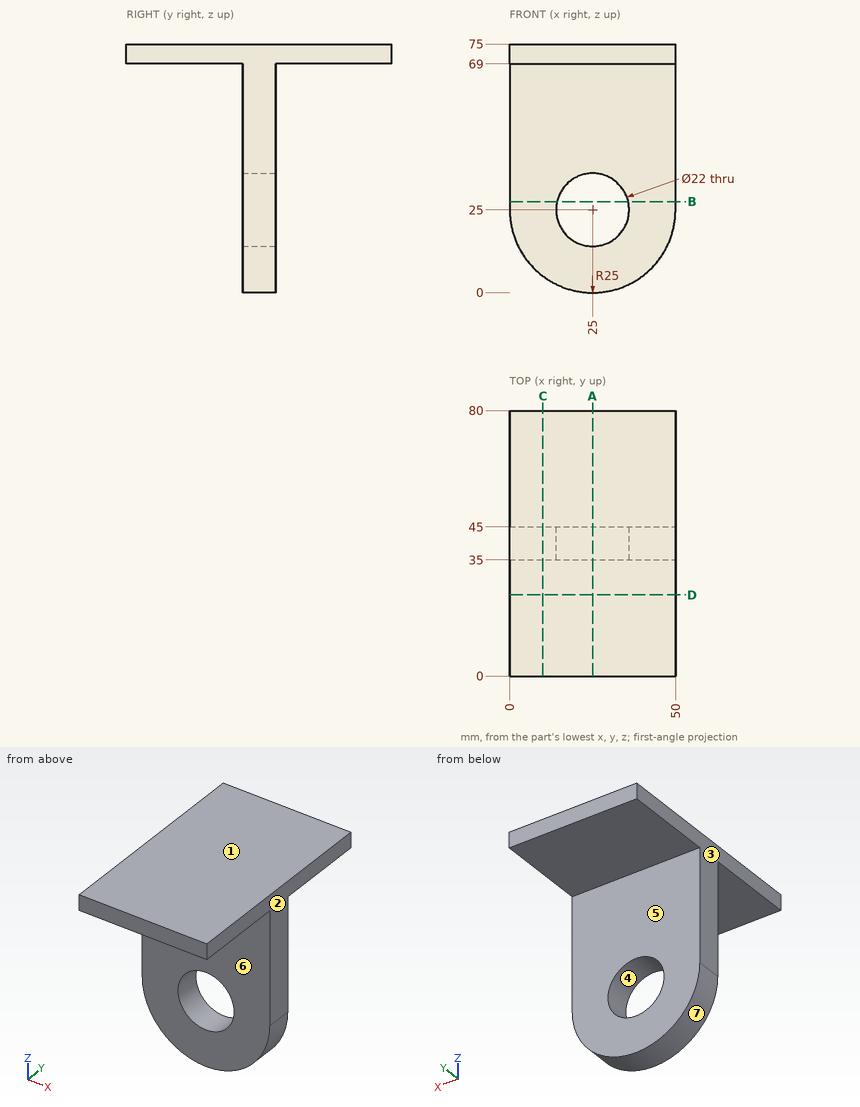
Input: dimensioned drawing with shaded views. Units: mm. Origin: part minimum x, y, z. A direction names the side the tool comes from. Round coordinates to 2 decimals unless told otherwise and drop trailing zeros. Order: outer loops, then holes, each group sorted by start corner. A loop starts at its lowest first (then second) coordinate and runs counter-clockwise, first axis right, second up. Notation, with made-up numbers: (0.5, 5) - (52.5, 5) arc R19 ccw to (52.5, 13) - close; hole circle Ø1 at (-22.75, 12.25). An arc over 180 degrees is marked (long way). Use CSV: the item, a comma, the result in double quotes. Start each with the question number.
Q1. Mould query, pull axis X, two halves, no side actions, for the marked faces 1, 2, 3 and 4. Classes: +X half, -X half, draft (parallel to the pull), parting line (faces both ways), or undercut.
Q2. Section query B-B (z = 27.5). Return loops of the section in (x, y), and give its area (3 significant figures).
Q3. Section query C-C (x = 10). Return loops of the section in (y, z), and give its area (3 significant figures).
Q4. Access query for the marked faces 5, 6 and 7. Directions: +Z, -Z, +X, -X, +Y, -Y. A direction counts if a zero-diameter tool reaches every point of the face in a straight line with its end or side. Return the directions, or none.
Q5. Material intervals for line 1 along Z through (x, y) = (25, 38); line 2 along Z through (x, y) = (33, 27.5); line 3 along Y through (x, z) = (31, 52), sorted ascending. Write a range as from..to.
Q6. First-contact query: pin 1 (2 mm diameter, centred on x = 23.5, y = 49, fed in from -Z); pin 2 (12 mm diameter, centred on x = 24, z = 58.5, fed in from -Y); pin 3 (10 mm diameter, centred on x = 29.5, z = 49, fed in from +Y). Flat tips, straight axial feed; report the tip coordinate or a pass-through.
Q7. Section query A-A (x = 25). Return loops of the section in (y, z).
Q8. Section query D-D (y = 24.5). Return loops of the section in (x, z).
Result set:
1,face 1,"draft"
1,face 2,"+X half"
1,face 3,"-X half"
1,face 4,"undercut"
2,outline,"(0, 35) - (14.29, 35) - (14.29, 45) - (0, 45) - close; (35.71, 35) - (50, 35) - (50, 45) - (35.71, 45) - close"
2,area,"286 mm2"
3,outline,"(0, 69) - (35, 69) - (35, 5) - (45, 5) - (45, 69) - (80, 69) - (80, 75) - (0, 75) - close"
3,area,"1,120 mm2"
4,face 5,"-Z, +X, -X, +Y"
4,face 6,"-Z, +X, -X, -Y"
4,face 7,"-Z, +Y, -Y"
5,line 1,"z = 0..14, 36..75"
5,line 2,"z = 69..75"
5,line 3,"y = 35..45"
6,pin 1,"stops at z = 69"
6,pin 2,"stops at y = 35"
6,pin 3,"stops at y = 45"
7,outline,"(0, 69) - (35, 69) - (35, 36) - (45, 36) - (45, 69) - (80, 69) - (80, 75) - (0, 75) - close; (35, 0) - (45, 0) - (45, 14) - (35, 14) - close"
8,outline,"(0, 69) - (50, 69) - (50, 75) - (0, 75) - close"
